Geometry: final body of the model. Coordinates: model frame, mm. Give positions to 0.01 mm unless a question says otherwise; leave off trailing zeros. Loops run counter-clockwise (first coordinate to the right, second up) from the corner with the lowest first, then second, coordinate; pieces in that order, holes last. Notation, with made-up numbers: (68.5, -14.5) - (82.5, -14.5) arc R28 cw to (82.5, 19.5) - close; hole circle Ø7 at (4.25, 33). An arc over 180 degrees is marked (long way). Use one line per item in the form item = value.
```python
from build123d import *

# Parameters (mm, degrees)
SKETCH1_R           = 2.5
BOSS_EXTRUDE1_DEPTH = 49.8
CUT_EXTRUDE2_DEPTH  = 3.7


with BuildPart() as part:
    # Sketch1 → Boss-Extrude1 (new body)
    with BuildSketch(Plane(origin=(0, 0, 0), x_dir=(0, 0, -1), z_dir=(1, 0, 0))):
        Circle(SKETCH1_R)
    extrude(amount=BOSS_EXTRUDE1_DEPTH)

    # Sketch3 → Cut-Extrude2 (cut)
    with BuildSketch(Plane.ZY):
        with BuildLine():
            Line((-2.537715508, -0.25), (-1.984313483, -0.25))
            ThreePointArc((-1.984313483, -0.25), (-1.931851653, -0.51763809), (-1.843465886, -0.775650391))
            Line((-1.843465886, -0.775650391), (-2.322726098, -1.052351403))
            ThreePointArc((-2.322726098, -1.052351403), (-2.463110857, -0.659988565), (-2.537715508, -0.25))
        make_face()
        with BuildLine():
            Line((-2.537715508, 0.25), (-1.984313483, 0.25))
            ThreePointArc((-1.984313483, 0.25), (-1.931851653, 0.51763809), (-1.843465886, 0.775650391))
            Line((-1.843465886, 0.775650391), (-2.322726098, 1.052351403))
            ThreePointArc((-2.322726098, 1.052351403), (-2.463110857, 0.659988565), (-2.537715508, 0.25))
        make_face()
        with BuildLine():
            Line((-2.072726098, 1.485364105), (-1.593465886, 1.208663093))
            ThreePointArc((-1.593465886, 1.208663093), (-1.414213562, 1.414213562), (-1.208663093, 1.593465886))
            Line((-1.208663093, 1.593465886), (-1.485364105, 2.072726098))
            ThreePointArc((-1.485364105, 2.072726098), (-1.803122292, 1.803122292), (-2.072726098, 1.485364105))
        make_face()
        with BuildLine():
            Line((-1.052351403, 2.322726098), (-0.775650391, 1.843465886))
            ThreePointArc((-0.775650391, 1.843465886), (-0.51763809, 1.931851653), (-0.25, 1.984313483))
            Line((-0.25, 1.984313483), (-0.25, 2.537715508))
            ThreePointArc((-0.25, 2.537715508), (-0.659988565, 2.463110857), (-1.052351403, 2.322726098))
        make_face()
        with BuildLine():
            Line((0.25, 2.537715508), (0.25, 1.984313483))
            ThreePointArc((0.25, 1.984313483), (0.51763809, 1.931851653), (0.775650391, 1.843465886))
            Line((0.775650391, 1.843465886), (1.052351403, 2.322726098))
            ThreePointArc((1.052351403, 2.322726098), (0.659988565, 2.463110857), (0.25, 2.537715508))
        make_face()
        with BuildLine():
            Line((1.485364105, 2.072726098), (1.208663093, 1.593465886))
            ThreePointArc((1.208663093, 1.593465886), (1.414213562, 1.414213562), (1.593465886, 1.208663093))
            Line((1.593465886, 1.208663093), (2.072726098, 1.485364105))
            ThreePointArc((2.072726098, 1.485364105), (1.803122292, 1.803122292), (1.485364105, 2.072726098))
        make_face()
        with BuildLine():
            Line((2.322726098, 1.052351403), (1.843465886, 0.775650391))
            ThreePointArc((1.843465886, 0.775650391), (1.931851653, 0.51763809), (1.984313483, 0.25))
            Line((1.984313483, 0.25), (2.537715508, 0.25))
            ThreePointArc((2.537715508, 0.25), (2.463110857, 0.659988565), (2.322726098, 1.052351403))
        make_face()
        with BuildLine():
            Line((2.537715508, -0.25), (1.984313483, -0.25))
            ThreePointArc((1.984313483, -0.25), (1.931851653, -0.51763809), (1.843465886, -0.775650391))
            Line((1.843465886, -0.775650391), (2.322726098, -1.052351403))
            ThreePointArc((2.322726098, -1.052351403), (2.463110857, -0.659988565), (2.537715508, -0.25))
        make_face()
        with BuildLine():
            Line((2.072726098, -1.485364105), (1.593465886, -1.208663093))
            ThreePointArc((1.593465886, -1.208663093), (1.414213562, -1.414213562), (1.208663093, -1.593465886))
            Line((1.208663093, -1.593465886), (1.485364105, -2.072726098))
            ThreePointArc((1.485364105, -2.072726098), (1.803122292, -1.803122292), (2.072726098, -1.485364105))
        make_face()
        with BuildLine():
            Line((1.052351403, -2.322726098), (0.775650391, -1.843465886))
            ThreePointArc((0.775650391, -1.843465886), (0.51763809, -1.931851653), (0.25, -1.984313483))
            Line((0.25, -1.984313483), (0.25, -2.537715508))
            ThreePointArc((0.25, -2.537715508), (0.659988565, -2.463110857), (1.052351403, -2.322726098))
        make_face()
        with BuildLine():
            Line((-0.25, -2.537715508), (-0.25, -1.984313483))
            ThreePointArc((-0.25, -1.984313483), (-0.51763809, -1.931851653), (-0.775650391, -1.843465886))
            Line((-0.775650391, -1.843465886), (-1.052351403, -2.322726098))
            ThreePointArc((-1.052351403, -2.322726098), (-0.659988565, -2.463110857), (-0.25, -2.537715508))
        make_face()
        with BuildLine():
            Line((-1.485364105, -2.072726098), (-1.208663093, -1.593465886))
            ThreePointArc((-1.208663093, -1.593465886), (-1.414213562, -1.414213562), (-1.593465886, -1.208663093))
            Line((-1.593465886, -1.208663093), (-2.072726098, -1.485364105))
            ThreePointArc((-2.072726098, -1.485364105), (-1.803122292, -1.803122292), (-1.485364105, -2.072726098))
        make_face()
    cut_extrude2 = extrude(amount=-CUT_EXTRUDE2_DEPTH, mode=Mode.SUBTRACT)

    # Mirror1: Cut-Extrude2 across plane
    add(cut_extrude2.mirror(Plane(origin=(24.9, 0, 0), x_dir=(0, 0, 1), z_dir=(1, 0, 0))), mode=Mode.SUBTRACT)


solid = part.part
```
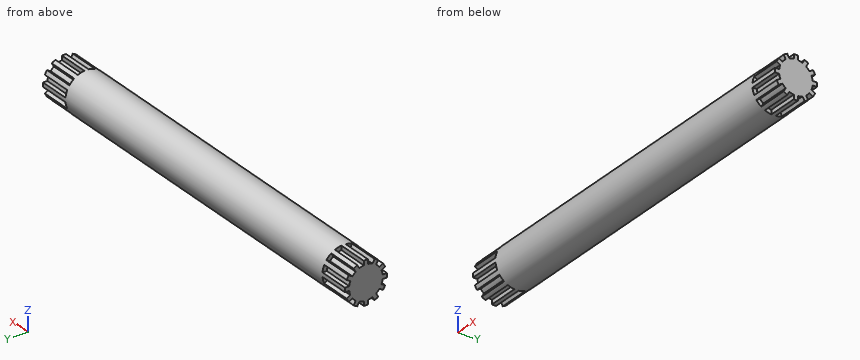
(1) Material intervals for L1, parallel to X at y = 1.65, z = 1.5; L2, parallel to Z at x = 39.5, y = 0.25; L3, parallel to Y at x = 21, z = 0.3, sorted ascending. Write a range as from..to.
Solution:
L1 = 3.7..46.1
L2 = -2.49..2.49
L3 = -2.48..2.48
(2) Pin query (flat end, axial travel): P1, Ø0.9, axis at y = -2, z = 2, coming from the +X side; P2, Ø2, axis at x = 40, z = -1.5, coming from the +Y side; P3, Ø1.5, axis at x = 14, z = -1.5, coming from the -Y side. Return the tip coordinate at first contact, or that it passes through.
Solution:
P1 = 46.1
P2 = 2.45
P3 = -2.38
(3) Cut plane A-A (x = 45). Return the cut outline in (y, z).
Solution:
outline = circle Ø5 at (0, 0)
